Answer from the drawing. Dimensions are ordinates in mm from the lowest x, y and z of the part. A direction names the side the tool comes from. Coordinates: 2 decimals unless noted, no trailing zeros. Order: outer loops, then holes, each group sorted by start corner. A loop starts at its lowest first (then second) coordinate and runs counter-clockwise, first axis right, second up.
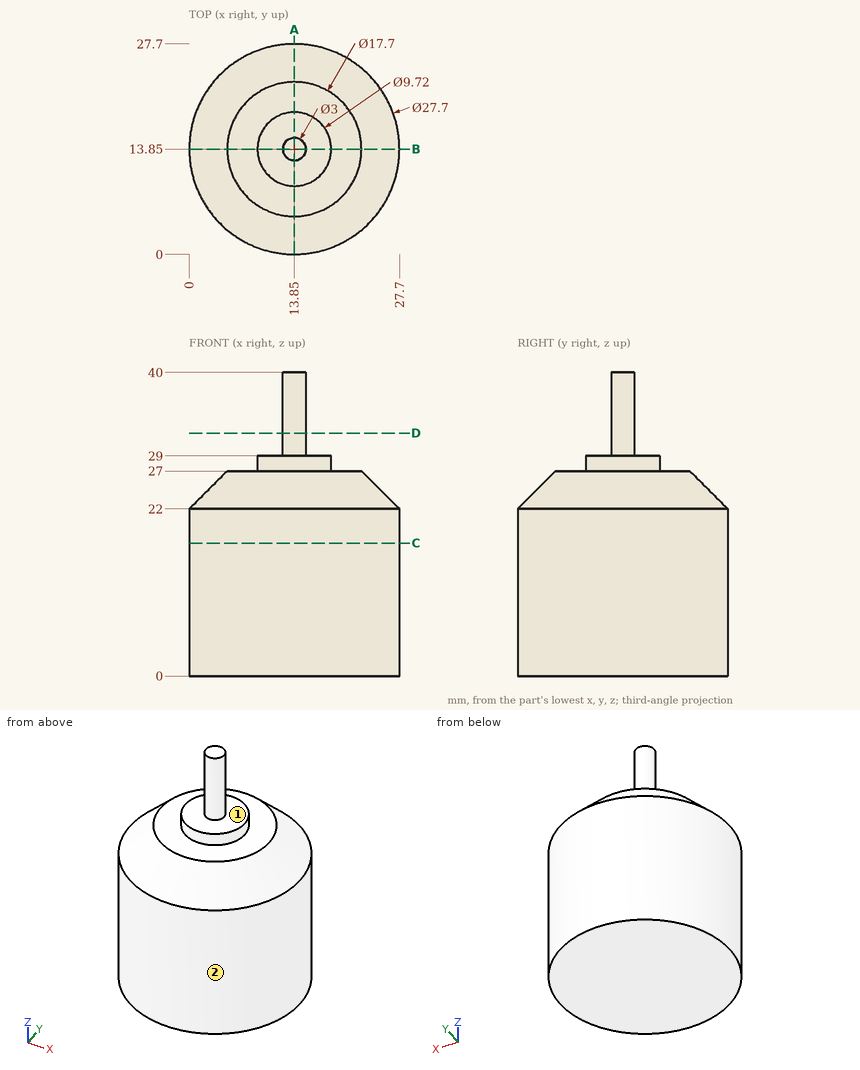
1. The part is cut by section C-C (z = 17.5). Determine the outline of the cut face in (x, y).
2. The part is cut by section A-A (x = 13.85). Determine the outline of the cut face in (y, z).
3. Flat-ended cylindrical pins translate along their axes: pin 1 (2 mm diameter, centred on x = 19.5, y = 8.5, fed in from +Z); pin 2 (1 mm diameter, centred on y = 15, z = 14, fed in from -X) (1 decimal); pin 3 (2 mm diameter, centred on x = 13.5, z = 25.5, fed in from +Y) (1 decimal). Find the tip coordinate at first contact, or state that the pin passes through.
4. The part is cut by section D-D (z = 32). Determine the outline of the cut face in (x, y).
5. For the marked faces 1 and 2, determine the directions among +Z, -Z, +X, -X, +Y, -Y from which every point of the face is accessible in a straight line to the end or side of a thin tool.
6. Consider probe 1 along Z at (x, y) = (8.25, 12.25); probe 2 along Y at (x, z) = (13.5, 10) (1 decimal); probe 3 along Z at (x, y) = (4.25, 22.75). Determine where each line is inside the solid, lowest interval first.
Worked out:
1. outline: circle Ø27.7 at (13.85, 13.85)
2. outline: (0, 0) - (27.7, 0) - (27.7, 22) - (22.7, 27) - (18.71, 27) - (18.71, 29) - (15.35, 29) - (15.35, 40) - (12.35, 40) - (12.35, 29) - (8.99, 29) - (8.99, 27) - (5, 27) - (0, 22) - close
3. pin 1: stops at z = 27
3. pin 2: stops at x = 0
3. pin 3: stops at y = 25.2
4. outline: circle Ø3 at (13.85, 13.85)
5. face 1: +Z
5. face 2: +Z, -Z
6. probe 1: z = 0 to 27
6. probe 2: y = 0 to 27.7
6. probe 3: z = 0 to 22.76
